```python
from build123d import *

# Parameters (mm, degrees)
F1_DEPTH = 63.5
F0_W     = 25.4674297452
F0_H     = 19.05
F2_DEPTH = 25.4
F3_DEPTH = 7.9375
F5_R     = 6.35


with BuildPart() as f1:
    # F0 (on Front) → F1 (new body, symmetric)
    with BuildSketch(Plane.XZ):
        Polygon((22.225, 9.525), (-41.275, 9.525), (-41.275, -9.525), (41.275, -9.525), (41.275, 9.525), align=None)
    extrude(amount=F1_DEPTH, both=True)

    # F0 (on Front) → F2 (join, symmetric)
    with BuildSketch(Plane.XZ):
        with BuildLine():
            Line((22.225, 27.0002), (22.225, 9.525))
            Line((22.225, 9.525), (41.275, 9.525))
            Line((41.275, 9.525), (41.275, 27.0002))
            ThreePointArc((41.275, 27.0002), (45.9246798487, 38.2255201513), (57.15, 42.8752))
            Line((57.15, 42.8752), (60.325, 42.8752))
            Line((60.325, 42.8752), (60.325, 61.9252))
            Line((60.325, 61.9252), (57.15, 61.9252))
            ThreePointArc((57.15, 61.9252), (32.4542956671, 51.6959043329), (22.225, 27.0002))
        make_face()
        with Locations((73.0587148726, 52.4002)):
            Rectangle(F0_W, F0_H)
    extrude(amount=F2_DEPTH, both=True)

    # F0 (on Front) → F3 (join, symmetric)
    with BuildSketch(Plane.XZ):
        with BuildLine():
            add(Edge.make_bspline(
                [(57.15, 61.9252), (15.1281916878, 62.2740810515), (-27.3216856892, 55.7221643058), (-41.6932850244, 18.0006596408), (-41.275, 9.525)],
                knots=[0, 0, 0, 0, 0.6030423214, 1, 1, 1, 1], degree=3))
            Line((-41.275, 9.525), (22.225, 9.525))
            Line((22.225, 9.525), (22.225, 27.0002))
            ThreePointArc((22.225, 27.0002), (32.4542956671, 51.6959043329), (57.15, 61.9252))
        make_face()
    extrude(amount=F3_DEPTH, both=True)

    # F0 (on Front) → F4 (revolve)
    with BuildSketch(Plane.XZ):
        Polygon((85.7924297452, 66.675), (85.7924297452, 61.9252), (85.7924297452, 42.8752), (85.7924297452, 38.1), (111.125, 38.1), (111.125, 66.675), align=None)
    revolve(axis=Axis((85.7924297452, 0, 52.3875), (0, 0, 1)))

    # F5
    f5_edges = [f1.edges().sort_by_distance(p)[0] for p in [
        (-41.275, -63.5, 0),
        (41.275, -63.5, 0),
        (41.275, 63.5, 0),
        (-41.275, 63.5, 0),
    ]]
    fillet(f5_edges, radius=F5_R)


solid = f1.part
```
Could you check a few things on this model? Use its own coordinates, in mm. A direction names the side the tool comes from. Coordinates: 2 decimals unless noted, no trailing zeros. Loops run counter-clockwise (first coordinate to the right, second up) from the corner with the lowest first, then second, coordinate; pieces in that order, holes last. Notation, with made-up numbers: M 67,85 L 76,85 A30 ccw 76,116 Z; hole C 84,46.25 d2. An arc over 180 degrees is marked long. Put each result on its own line as item: value. Start each with the question number.
(1) Will these pins go through, and if not, where does the flat tip stop? P1, Ø11, axis at y = -21, z = 18, coming from the +X side (3 decimals); P2, Ø1, axis at y = -12, z = -1.5, coming from the -X side (3 decimals); P3, Ø8, axis at x = 41, y = 13, coming from the +Z side; P4, Ø1, axis at y = -44.5, z = 11.5, coming from the -X side.
(2) Suppose I cut it at B-B on y = -49. Please give me the cut outline in (x, z) (3 decimals), then the cut area to 3 significant figures.
(3) I need wall thicknesses on line 1 (Z direction, x = -17, y = -27.5) (3 decimals); line 2 (Y direction, x = 49.5, z = 48.5); line 3 (Y direction, x = -1.5, z = 34). Which ranges of each line are inside material? Lowest first, please. Write a range as from..to.
(4) Suppose I cut it at C-C on x = 64. Please give me the cut outline in (y, z) (3 decimals), then the cut area to 3 significant figures.
(5) Suppose I cut it at A-A on z = 3. Please give me the cut outline in (x, y) (3 decimals).
(6) For faces 1 (the face through (-4, -7.938, 36)), 2 (the face through (41.275, -1, 4)), 3 (the face through (60, 0, 61.925)), 4 (the face through (47, 25.4, 42)), which set-ups out of +Z, -Z, +X, -X, +Y, -Y let a thin tool reach every point of the face, with its end or its side?
Solutions:
1. P1: stops at x = 41.275
1. P2: stops at x = -41.275
1. P3: stops at z = 59.74
1. P4: passes through
2. outline: M -41.275,-9.525 L 41.275,-9.525 L 41.275,9.525 L -41.275,9.525 Z
2. area: 1,570 mm2
3. line 1: z = -9.525..9.525
3. line 2: y = -25.4..25.4
3. line 3: y = -7.94..7.94
4. outline: M -25.4,42.875 L -12.916,42.875 L -12.916,38.1 L 12.916,38.1 L 12.916,42.875 L 25.4,42.875 L 25.4,61.925 L 12.916,61.925 L 12.916,66.675 L -12.916,66.675 L -12.916,61.925 L -25.4,61.925 Z
4. area: 1,210 mm2
5. outline: M -41.275,-57.15 A6.35 ccw -34.925,-63.5 L 34.925,-63.5 A6.35 ccw 41.275,-57.15 L 41.275,57.15 A6.35 ccw 34.925,63.5 L -34.925,63.5 A6.35 ccw -41.275,57.15 Z
6. face 1: +Z, -X, -Y
6. face 2: -Z, +X, +Y, -Y
6. face 3: +Z, -X
6. face 4: +Z, +X, -X, +Y
